Model file for the job. Use its own axes, mm. Face numbers are marked on the shaded views. A direction names the side the tool comes from. Coordinates: 2 decimals unless noted, no trailing zeros. Order: outer loops, then holes, each group sorted by start corner. A loop starts at its lowest first (then second) coordinate and runs counter-clockwise, first axis right, second up.
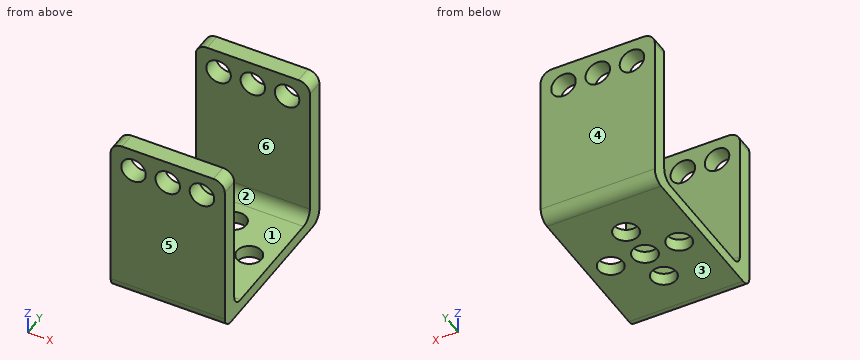
Autodesk Inventor part; units mm, degrees
ref_plane "YZ Plane" through (0, 0, 0) normal (1, 0, 0) x (0, 1, 0)
ref_plane "XZ Plane" through (0, 0, 0) normal (0, 1, 0) x (-1, 0, 0)
ref_plane "XY Plane" through (0, 0, 0) normal (0, 0, 1) x (1, 0, 0)
sketch "Esquisse5" plane through (0, 0, 0) normal (0, 0, 1) x (1, 0, 0)
  line L0 (0, 0) -> (20, 0)
  line L1 (20, 0) -> (20, 30)
  line L2 (20, 30) -> (0, 30)
  line L3 (0, 30) -> (0, 0)
  line L4 (10, 0) -> (10, 30) construction
  circle A0 centre (10, 9) radius 2.15
  circle A1 centre (10, 15) radius 2.15
  circle A2 centre (10, 21) radius 2.15
  line L5 (10, 15) -> (20, 15) construction
  circle A3 centre (16, 15) radius 2.15
  circle A4 centre (4, 15) radius 2.15
  circle A5 centre (10, 15) radius 2.15
  dimension "d61" = 20
  dimension "d62" = 30
  dimension "d64" = 4.3
  dimension "d67" = 6
  dimension "d74" = 6
  dimension "d77" = 6
extrude "Extrusion5" add sketch "Esquisse5" along normal blind 2.2
sketch "Esquisse9" plane through (0, 0, 2.2) normal (0, 0, 1) x (1, 0, 0)
  line L0 (20, 0) -> (20, 30) construction
  line L1 (0, 30) -> (0, 0) construction
  line L2 (0, 30) -> (20, 30)
  line L3 (20, 30) -> (20, 27)
  line L4 (20, 27) -> (0, 27)
  line L5 (0, 27) -> (0, 30)
  line L6 (0, 15) -> (20, 15) construction
  line L7 (20, 0) -> (0, 0) construction
  line L8 (0, 0) -> (20, 0)
  line L9 (20, 0) -> (20, 3)
  line L10 (20, 3) -> (0, 3)
  line L11 (0, 3) -> (0, 0)
  dimension "d102" = 3
extrude "Extrusion9" add sketch "Esquisse9" along normal blind 27
sketch "Esquisse10" plane through (0, 0, 0) normal (0, -1, 0) x (1, 0, 0)
  line L0 (0, 0) -> (20, 0) construction
  line L1 (20, 0) -> (20, 29.2) construction
  line L2 (0, 29.2) -> (20, 29.2) construction
  line L3 (10, 29.2) -> (10, 0) construction
  circle A0 centre (10, 25.2) radius 2.15
  line L4 (10, 25.2) -> (20, 25.2) construction
  circle A1 centre (16, 25.2) radius 2.15
  circle A2 centre (4, 25.2) radius 2.15
  circle A3 centre (10, 25.2) radius 2.15
  dimension "d105" = 4
  dimension "d106" = 4.3
  dimension "d109" = 6
  dimension "d112" = 6
extrude "Extrusion10" cut sketch "Esquisse10" against normal through all
fillet "Congé6" radius 2 8 edges at (10, 0, 0) (10, 3, 2.2) (10, 27, 2.2) (0, 28.5, 29.2) (20, 28.5, 29.2) (20, 1.5, 29.2) (0, 1.5, 29.2) (10, 30, 0)
equation "\"d64\" = Holes"
equation "\"d80\" = Depth"
equation "\"d106\" = Holes"
equation "\"Depth\" = 2.2"
equation "\"Holes\" = 4.3"
equation "\"Height\" = 0"
equation "\"Rounding\" = 7"
equation "\"BackLegUpperBoneLength\" = 17"
properties part number "BackLegUpperUpperBone"
Q1. Cut at C-C, the plane x = 10. Count the separate pieces of the cut face and the enclosed holes in it, plus the area to 3 significant figures.
Established:
separate pieces: 6
enclosed holes: 0
area: 174 mm2
Q2. Drop flat-ended pins along their axis: P1, Ø3, axis at y = 5.5, z = 16, coming from the -X side; P2, Ø3, axis at x = 7.5, y = 11.5, coming from the +Z side. Give the stop position or say it passes through.
Established:
P1: passes through
P2: stops at z = 2.2
Q3. Mould opens along Y. For the marked faces 1, 2, 3 and 4 say: pulls with the +Y half, pulls with the -Y half, needs draft (parallel to the pull), parting line crosses it, or undercut.
Established:
face 1: undercut
face 2: undercut
face 3: needs draft
face 4: pulls with the +Y half
Q4. Cut at B-B, the plane z = 8. List the corners of the cut face in (x, y).
Established:
outline: (0, 0) - (20, 0) - (20, 3) - (0, 3) - close; (0, 27) - (20, 27) - (20, 30) - (0, 30) - close
Q5. Probe line 1 (Z direction, x = 4, y = 2.25); line 2 (Y direction, x = 6.75, z = 25.5); line 3 (Y direction, x = 10, z = 1.2). List the from-to ranges inside material, lowest first.
Established:
line 1: z = 0 to 23.05, 27.35 to 29.2
line 2: y = 0 to 3, 27 to 30
line 3: y = 0.17 to 6.85, 11.15 to 12.85, 17.15 to 18.85, 23.15 to 29.83
Q6. Which spindle directions (+Z, -Z, +X, -X, +Y, -Y) get a long thin tool onto all of the face, cutting with end or side? Do the marked faces 5 and 6. Say none if no direction does.
Established:
face 5: +Z, -Z, +X, -X, -Y
face 6: +Z, +X, -X
Q7. Cut at A-A, the plane y = 9. List the corners of the cut face in (x, z).
Established:
outline: (0, 0) - (7.85, 0) - (7.85, 2.2) - (0, 2.2) - close; (12.15, 0) - (20, 0) - (20, 2.2) - (12.15, 2.2) - close
